from build123d import *

# Parameters (mm, degrees)
SKETCH1_W           = 110
SKETCH1_H           = 82
BOSS_EXTRUDE1_DEPTH = 6.35
CUT_EXTRUDE1_REACH  = 8.35
SKETCH2_W           = 82
SKETCH2_H           = 72
SKETCH3_W           = 110
SKETCH3_H           = 97.464272111
BOSS_EXTRUDE2_DEPTH = 6.35
CUT_EXTRUDE2_REACH  = 8.35
FILLET1_R           = 5
CUT_EXTRUDE3_REACH  = 8.35
SKETCH5_R           = 2.5019
SKETCH5_R_2         = 4.25


with BuildPart() as part:
    # Sketch1 → Boss-Extrude1 (new body)
    with BuildSketch(Plane.XY):
        with Locations((55, 41)):
            Rectangle(SKETCH1_W, SKETCH1_H)
    extrude(amount=BOSS_EXTRUDE1_DEPTH)

    # Sketch2 → Cut-Extrude1 (cut, up to next)
    with BuildSketch(Plane.XY.offset(6.35), mode=Mode.PRIVATE) as cut_extrude1_sk1:
        with Locations((55, 41)):
            Rectangle(SKETCH2_W, SKETCH2_H)
    cut_extrude1_tool1 = extrude(cut_extrude1_sk1.sketch, amount=-CUT_EXTRUDE1_REACH, mode=Mode.PRIVATE) & part.part
    add(cut_extrude1_tool1.solids().sort_by_distance((55, 41, 6.35))[0], mode=Mode.SUBTRACT)

    # Sketch3 → Boss-Extrude2 (add)
    with BuildSketch(Plane.XY.offset(6.35)):
        with Locations((55, -48.732136055)):
            Rectangle(SKETCH3_W, SKETCH3_H)
    extrude(amount=-BOSS_EXTRUDE2_DEPTH)

    # Sketch4 → Cut-Extrude2 (cut, up to next)
    with BuildSketch(Plane.XY.offset(6.35), mode=Mode.PRIVATE) as cut_extrude2_sk1:
        with BuildLine():
            Line((10, -69.464272111), (35, -69.464272111))
            ThreePointArc((35, -69.464272111), (40.5, -74.964272111), (35, -80.464272111))
            Line((35, -80.464272111), (10, -80.464272111))
            ThreePointArc((10, -80.464272111), (4.5, -74.964272111), (10, -69.464272111))
        make_face()
    cut_extrude2_tool1 = extrude(cut_extrude2_sk1.sketch, amount=-CUT_EXTRUDE2_REACH, mode=Mode.PRIVATE) & part.part
    add(cut_extrude2_tool1.solids().sort_by_distance((22.5, -74.964272, 6.35))[0], mode=Mode.SUBTRACT)
    # Sketch4 → Cut-Extrude2 (cut, up to next)
    with BuildSketch(Plane.XY.offset(6.35), mode=Mode.PRIVATE) as cut_extrude2_sk2:
        with BuildLine():
            Line((100, -69.464272111), (75, -69.464272111))
            ThreePointArc((75, -69.464272111), (69.5, -74.964272111), (75, -80.464272111))
            Line((75, -80.464272111), (100, -80.464272111))
            ThreePointArc((100, -80.464272111), (105.5, -74.964272111), (100, -69.464272111))
        make_face()
    cut_extrude2_tool2 = extrude(cut_extrude2_sk2.sketch, amount=-CUT_EXTRUDE2_REACH, mode=Mode.PRIVATE) & part.part
    add(cut_extrude2_tool2.solids().sort_by_distance((87.5, -74.964272, 6.35))[0], mode=Mode.SUBTRACT)
    # Sketch4 → Cut-Extrude2 (cut, up to next)
    with BuildSketch(Plane.XY.offset(6.35), mode=Mode.PRIVATE) as cut_extrude2_sk3:
        with BuildLine():
            Line((10, -35.464272111), (35, -35.464272111))
            ThreePointArc((35, -35.464272111), (40.5, -29.964272111), (35, -24.464272111))
            Line((35, -24.464272111), (10, -24.464272111))
            ThreePointArc((10, -24.464272111), (4.5, -29.964272111), (10, -35.464272111))
        make_face()
    cut_extrude2_tool3 = extrude(cut_extrude2_sk3.sketch, amount=-CUT_EXTRUDE2_REACH, mode=Mode.PRIVATE) & part.part
    add(cut_extrude2_tool3.solids().sort_by_distance((22.5, -29.964272, 6.35))[0], mode=Mode.SUBTRACT)
    # Sketch4 → Cut-Extrude2 (cut, up to next)
    with BuildSketch(Plane.XY.offset(6.35), mode=Mode.PRIVATE) as cut_extrude2_sk4:
        with BuildLine():
            Line((100, -35.464272111), (75, -35.464272111))
            ThreePointArc((75, -35.464272111), (69.5, -29.964272111), (75, -24.464272111))
            Line((75, -24.464272111), (100, -24.464272111))
            ThreePointArc((100, -24.464272111), (105.5, -29.964272111), (100, -35.464272111))
        make_face()
    cut_extrude2_tool4 = extrude(cut_extrude2_sk4.sketch, amount=-CUT_EXTRUDE2_REACH, mode=Mode.PRIVATE) & part.part
    add(cut_extrude2_tool4.solids().sort_by_distance((87.5, -29.964272, 6.35))[0], mode=Mode.SUBTRACT)

    # Fillet1
    fillet1_edges = [part.edges().sort_by_distance(p)[0] for p in [
        (110, -97.464272111, 3.175),
        (0, -97.464272111, 3.175),
        (0, 82, 3.175),
        (110, 82, 3.175),
    ]]
    fillet(fillet1_edges, radius=FILLET1_R)

    # Sketch5 → Cut-Extrude3 (cut, up to next)
    with BuildSketch(Plane.XY.offset(6.35), mode=Mode.PRIVATE) as cut_extrude3_sk1:
        with Locations((7.2988, 11.0026)):
            Circle(SKETCH5_R)
    cut_extrude3_tool1 = extrude(cut_extrude3_sk1.sketch, amount=-CUT_EXTRUDE3_REACH, mode=Mode.PRIVATE) & part.part
    add(cut_extrude3_tool1.solids().sort_by_distance((7.2988, 11.0026, 6.35))[0], mode=Mode.SUBTRACT)
    # Sketch5 → Cut-Extrude3 (cut, up to next)
    with BuildSketch(Plane.XY.offset(6.35), mode=Mode.PRIVATE) as cut_extrude3_sk2:
        with Locations((7.2988, 70.9974)):
            Circle(SKETCH5_R)
    cut_extrude3_tool2 = extrude(cut_extrude3_sk2.sketch, amount=-CUT_EXTRUDE3_REACH, mode=Mode.PRIVATE) & part.part
    add(cut_extrude3_tool2.solids().sort_by_distance((7.2988, 70.9974, 6.35))[0], mode=Mode.SUBTRACT)
    # Sketch5 → Cut-Extrude3 (cut, up to next)
    with BuildSketch(Plane.XY.offset(6.35), mode=Mode.PRIVATE) as cut_extrude3_sk3:
        with Locations((102.7012, 70.9974)):
            Circle(SKETCH5_R)
    cut_extrude3_tool3 = extrude(cut_extrude3_sk3.sketch, amount=-CUT_EXTRUDE3_REACH, mode=Mode.PRIVATE) & part.part
    add(cut_extrude3_tool3.solids().sort_by_distance((102.7012, 70.9974, 6.35))[0], mode=Mode.SUBTRACT)
    # Sketch5 → Cut-Extrude3 (cut, up to next)
    with BuildSketch(Plane.XY.offset(6.35), mode=Mode.PRIVATE) as cut_extrude3_sk4:
        with Locations((102.7012, 11.0026)):
            Circle(SKETCH5_R)
    cut_extrude3_tool4 = extrude(cut_extrude3_sk4.sketch, amount=-CUT_EXTRUDE3_REACH, mode=Mode.PRIVATE) & part.part
    add(cut_extrude3_tool4.solids().sort_by_distance((102.7012, 11.0026, 6.35))[0], mode=Mode.SUBTRACT)
    # Sketch5 → Cut-Extrude3 (cut, up to next)
    with BuildSketch(Plane.XY.offset(6.35), mode=Mode.PRIVATE) as cut_extrude3_sk5:
        with Locations((7.2988, 41)):
            Circle(SKETCH5_R_2)
    cut_extrude3_tool5 = extrude(cut_extrude3_sk5.sketch, amount=-CUT_EXTRUDE3_REACH, mode=Mode.PRIVATE) & part.part
    add(cut_extrude3_tool5.solids().sort_by_distance((7.2988, 41, 6.35))[0], mode=Mode.SUBTRACT)
    # Sketch5 → Cut-Extrude3 (cut, up to next)
    with BuildSketch(Plane.XY.offset(6.35), mode=Mode.PRIVATE) as cut_extrude3_sk6:
        with Locations((102.7012, 41)):
            Circle(SKETCH5_R_2)
    cut_extrude3_tool6 = extrude(cut_extrude3_sk6.sketch, amount=-CUT_EXTRUDE3_REACH, mode=Mode.PRIVATE) & part.part
    add(cut_extrude3_tool6.solids().sort_by_distance((102.7012, 41, 6.35))[0], mode=Mode.SUBTRACT)


solid = part.part
Build history of the part. All positions in model axes, mm. A direction names the side the tool comes from. Round coordinates to 2 decimals unless told otherwise and drop trailing zeros. Write each loop counter-clockwise with the first axis right and the second up, starting at its lowest first coordinate (ties: lowest second). Pieces come first, ordered by that corner, then holes. Notation, with made-up numbers: M 3.25,24.5 L 57.25,24.5 A13 cw 57.25,37.5 Z; hole C 12.25,80 d4. An arc over 180 degrees is marked long. Answer in a Markdown table with one row per item.
1. Saw through at B-B (x = 31). List the corners of the cut face in (y, z).
Geometry check:
| item | result |
|---|---|
| outline | M -97.46,0 L -80.46,0 L -80.46,6.35 L -97.46,6.35 Z; M -69.46,0 L -35.46,0 L -35.46,6.35 L -69.46,6.35 Z; M -24.46,0 L 5,0 L 5,6.35 L -24.46,6.35 Z; M 77,0 L 82,0 L 82,6.35 L 77,6.35 Z |
2. Saw through at D-D (z = 4). State how many separate pieces and enclosed holes the cut face has, and give its area (3 significant figures).
Geometry check:
| item | result |
|---|---|
| separate pieces | 1 |
| enclosed holes | 11 |
| area | 12,100 mm2 |
3. Flat gauge pin, fed straight in: P1, Ø5, axis at x = 102.7, y = 41, coming from the -Z side. Where does the tip first touch, or does it go through?
Geometry check:
| item | result |
|---|---|
| P1 | through |
4. Saw through at C-C (x = 102). List the corners of the cut face in (y, z), and give its area (3 significant figures).
Geometry check:
| item | result |
|---|---|
| outline | M -97.46,0 L -80.09,0 L -80.09,6.35 L -97.46,6.35 Z; M -69.84,0 L -35.09,0 L -35.09,6.35 L -69.84,6.35 Z; M -24.84,0 L 8.6,0 L 8.6,6.35 L -24.84,6.35 Z; M 13.4,0 L 36.81,0 L 36.81,6.35 L 13.4,6.35 Z; M 45.19,0 L 68.6,0 L 68.6,6.35 L 45.19,6.35 Z; M 73.4,0 L 82,0 L 82,6.35 L 73.4,6.35 Z |
| area | 895 mm2 |
5. Mould opens along X. For faces 1 (the face through (0, -9, 3)), 2 (the face through (108, 81, 3)), 3 (the face through (3.93, 38.41, 3.22)) say: +X half, -X half, draft (parallel to the pull), parting line (faces both ways), or undercut.
Geometry check:
| item | result |
|---|---|
| face 1 | -X half |
| face 2 | +X half |
| face 3 | undercut |
6. Saw through at A-A (y = 41). List the corners of the cut face in (x, z), and give its area (4 significant figures).
Geometry check:
| item | result |
|---|---|
| outline | M 0,0 L 3.05,0 L 3.05,6.35 L 0,6.35 Z; M 11.55,0 L 14,0 L 14,6.35 L 11.55,6.35 Z; M 96,0 L 98.45,0 L 98.45,6.35 L 96,6.35 Z; M 106.95,0 L 110,0 L 110,6.35 L 106.95,6.35 Z |
| area | 69.85 mm2 |
7. Which spindle directions (+Z, -Z, +X, -X, +Y, -Y) get a long thin tool onto all of the face, cutting with end or side? Do faces 4 (the face through (4.5, -75.1, 3.2)), 5 (the face through (54, -46, 0)). Say none if no direction does.
Geometry check:
| item | result |
|---|---|
| face 4 | +Z, -Z |
| face 5 | -Z, +X, -X, +Y, -Y |
8. Probe L1, parallel to Y at x = 24, z = 4.5; L2, parallel to Y at x = 43, z = 6; L3, parallel to Y at x = 38, z = 2. List the from-to ranges inside material, lowest first. Write a range as [from, to].
Geometry check:
| item | result |
|---|---|
| L1 | [-97.46, -80.46], [-69.46, -35.46], [-24.46, 5], [77, 82] |
| L2 | [-97.46, 5], [77, 82] |
| L3 | [-97.46, -79.57], [-70.35, -34.57], [-25.35, 5], [77, 82] |
